Job drawing, mm, ordinate dimensions from the low corner. One solid piece. Round coordinates to 2 decimals unless told otherwise and drop trailing zeros. Loops run counter-clockwise (first coordinate to the right, second up) from the corner with the lowest first, then second, coordinate; pieces in that order, holes last. Notation, with made-up numbers: M 73.5,69 L 77.5,69 A21 cw 77.5,89 Z; hole C 42.25,51 d10. An arc over 180 degrees is marked long. Use one line per item in the form item = value. Start each with the question number.
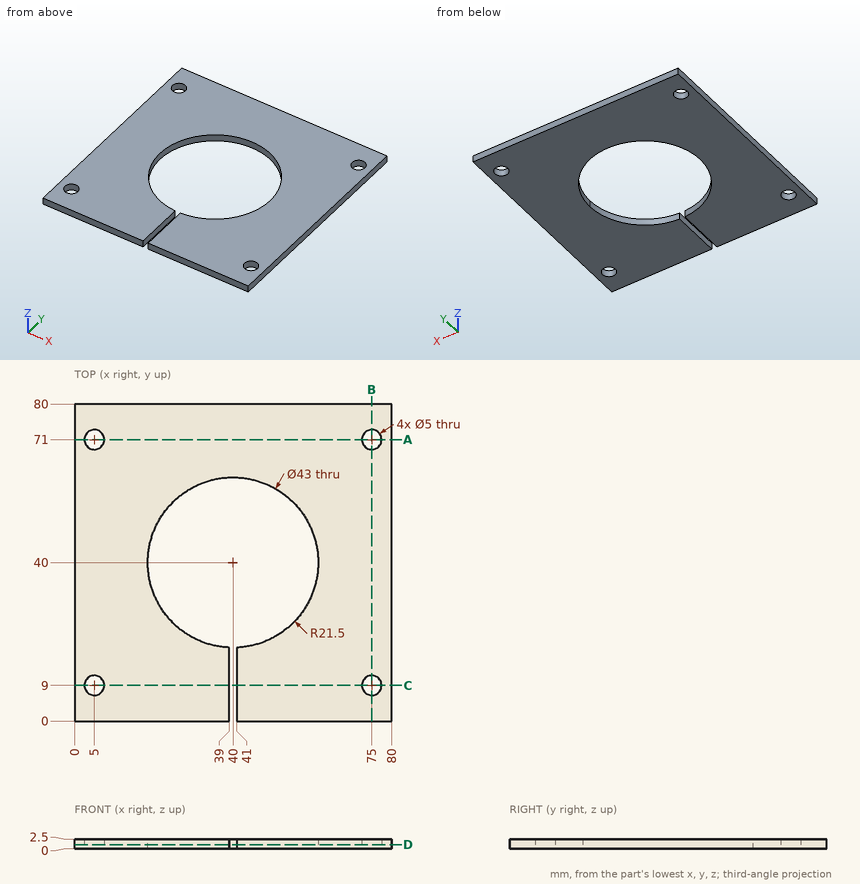
Q1. Saw through at C-C (y = 9). Give the cut face in (x, z).
Q2. Drop a flat-ended pin along its axis: P1, Ø1, axis at y = 51, z = 0.5, coming from the -X side. Give the stop position or say it passes through.
Q3. Saw through at B-B (x = 75). Give the cut face in (y, z), and give its area (3 significant figures).
Q4. Saw through at D-D (z = 1.1). Give the cut face in (x, y).
Q5. Saw through at A-A (y = 71). Give the cut face in (x, z).
Q6. Wall check: probe 1 along Y at (x, z) = (75, 0.75); probe 2 along X at (y, z) = (71, 1); probe 3 along Y at (x, z) = (74, 1.5). Give the ranges that are in metal, low to high.
Filled in:
q1.outline = M 0,0 L 2.5,0 L 2.5,2.5 L 0,2.5 Z; M 7.5,0 L 39,0 L 39,2.5 L 7.5,2.5 Z; M 41,0 L 72.5,0 L 72.5,2.5 L 41,2.5 Z; M 77.5,0 L 80,0 L 80,2.5 L 77.5,2.5 Z
q2.P1 = 0
q3.outline = M 0,0 L 6.5,0 L 6.5,2.5 L 0,2.5 Z; M 11.5,0 L 68.5,0 L 68.5,2.5 L 11.5,2.5 Z; M 73.5,0 L 80,0 L 80,2.5 L 73.5,2.5 Z
q3.area = 175 mm²
q4.outline = M 0,0 L 39,0 L 39,18.52 A21.5 cw long 41,18.52 L 41,0 L 80,0 L 80,80 L 0,80 Z; hole C 5,9 d5; hole C 5,71 d5; hole C 75,9 d5; hole C 75,71 d5
q5.outline = M 0,0 L 2.5,0 L 2.5,2.5 L 0,2.5 Z; M 7.5,0 L 72.5,0 L 72.5,2.5 L 7.5,2.5 Z; M 77.5,0 L 80,0 L 80,2.5 L 77.5,2.5 Z
q6.probe_1 = 0 to 6.5, 11.5 to 68.5, 73.5 to 80
q6.probe_2 = 0 to 2.5, 7.5 to 72.5, 77.5 to 80
q6.probe_3 = 0 to 6.71, 11.29 to 68.71, 73.29 to 80
